```python
from build123d import *

# Parameters (mm, degrees)
SKETCH1_W           = 25.4
SKETCH1_H           = 25.4
SKETCH1_W_2         = 22.225
SKETCH1_H_2         = 22.225
BOSS_EXTRUDE1_DEPTH = 234.95
FILLET1_R           = 2.54
SKETCH2_R           = 3.175
CUT_EXTRUDE1_DEPTH  = 238.560919126
SKETCH3_R           = 1.7
CUT_EXTRUDE2_DEPTH  = 2.54


with BuildPart() as part:
    # Sketch1 → Boss-Extrude1 (new body)
    with BuildSketch(Plane.XY):
        with Locations((-11.559591837, -1.275183673)):
            Rectangle(SKETCH1_W, SKETCH1_H)
        with Locations((-11.559591837, -1.275183673)):
            Rectangle(SKETCH1_W_2, SKETCH1_H_2, mode=Mode.SUBTRACT)
    extrude(amount=BOSS_EXTRUDE1_DEPTH)

    # Fillet1
    fillet1_edges = [part.edges().sort_by_distance(p)[0] for p in [
        (-24.259591837, 11.424816327, 117.475),
        (1.140408163, 11.424816327, 117.475),
        (1.140408163, -13.975183673, 117.475),
        (-24.259591837, -13.975183673, 117.475),
    ]]
    fillet(fillet1_edges, radius=FILLET1_R)

    # Sketch2 → Cut-Extrude1 (cut, through all)
    with BuildSketch(Plane(origin=(0, 11.424816327, 0), x_dir=(1, 0, 0), z_dir=(0, 1, 0))):
        with Locations(Location((-11.559591837, -12.7, 0), (0, 0, 270))):
            Circle(SKETCH2_R)
        with Locations(Location((-11.559591837, -38.1, 0), (0, 0, 270))):
            Circle(SKETCH2_R)
    extrude(amount=-CUT_EXTRUDE1_DEPTH, mode=Mode.SUBTRACT)

    # Sketch3 → Cut-Extrude2 (cut)
    with BuildSketch(Plane(origin=(0, 11.424816327, 0), x_dir=(1, 0, 0), z_dir=(0, 1, 0))):
        with Locations(Location((-6.745071652, -209.51091592, 0), (0, 0, 270))):
            Circle(SKETCH3_R)
        with Locations(Location((-4.172146269, -206.096528614, 0), (0, 0, 270))):
            Circle(SKETCH3_R)
        with Locations(Location((-3.921994623, -221.549522883, 0), (0, 0, 270))):
            Circle(SKETCH3_R)
        with BuildLine():
            Line((-15.016431655, -223.31216962), (-17.859841481, -227.085501905))
            ThreePointArc((-17.859841481, -227.085501905), (-20.240607387, -227.420096733), (-20.575202215, -225.039330826))
            Line((-20.575202215, -225.039330826), (-17.731792389, -221.265998541))
            ThreePointArc((-17.731792389, -221.265998541), (-15.351026483, -220.931403713), (-15.016431655, -223.31216962))
        make_face()
        with BuildLine():
            Line((-18.594632259, -208.581648392), (-17.777811336, -209.185849998))
            ThreePointArc((-17.777811336, -209.185849998), (-17.422050667, -211.563545173), (-19.799745842, -211.919305842))
            Line((-19.799745842, -211.919305842), (-20.616566765, -211.315104237))
            ThreePointArc((-20.616566765, -211.315104237), (-20.972327435, -208.937409062), (-18.594632259, -208.581648392))
        make_face()
    extrude(amount=-CUT_EXTRUDE2_DEPTH, mode=Mode.SUBTRACT)


solid = part.part
```
The listing builds one solid part. Answer for the finished solid, in the listing's coordinates (mm). A direction names the side the tool comes from. Give positions to 0.01 mm unless a question says otherwise; leave off trailing zeros. Order: outer loops, then holes, each group sorted by start corner. A loop starts at its lowest first (then second) coordinate and runs counter-clockwise, first axis right, second up.
Item 1: The part is cut by section C-C, the plane z = 109. Give the vertices of the cut face in (x, y), and give its area (3 significant figures).
From the geometry:
outline: (-24.26, -11.44) arc R2.54 ccw to (-21.72, -13.98) - (-1.4, -13.98) arc R2.54 ccw to (1.14, -11.44) - (1.14, 8.88) arc R2.54 ccw to (-1.4, 11.42) - (-21.72, 11.42) arc R2.54 ccw to (-24.26, 8.88) - close; hole (-22.67, -12.39) - (-0.45, -12.39) - (-0.45, 9.84) - (-22.67, 9.84) - close
area: 146 mm2
Item 2: The part is cut by section B-B, the plane y = -6.25. Give the vertices of the cut face in (x, z), and give its area (3 significant figures).
From the geometry:
outline: (-24.26, 0) - (-22.67, 0) - (-22.67, 234.95) - (-24.26, 234.95) - close; (-0.45, 0) - (1.14, 0) - (1.14, 234.95) - (-0.45, 234.95) - close
area: 746 mm2
Item 3: Given pin 1 Ø5.5 at (x, z) = (-11.56, 12.7) entering from +Y, flat-ended and moving along its own axis, determine where the tip first touches the part or whether it passes through.
From the geometry:
pin 1: passes through
Item 4: The part is cut by section A-A, the plane z = 38.1. Give the vertices of the cut face in (x, y).
From the geometry:
outline: (-24.26, -11.44) arc R2.54 ccw to (-21.72, -13.98) - (-14.73, -13.98) - (-14.73, -12.39) - (-22.67, -12.39) - (-22.67, 9.84) - (-14.73, 9.84) - (-14.73, 11.42) - (-21.72, 11.42) arc R2.54 ccw to (-24.26, 8.88) - close; (-8.38, -13.98) - (-1.4, -13.98) arc R2.54 ccw to (1.14, -11.44) - (1.14, 8.88) arc R2.54 ccw to (-1.4, 11.42) - (-8.38, 11.42) - (-8.38, 9.84) - (-0.45, 9.84) - (-0.45, -12.39) - (-8.38, -12.39) - close
Item 5: Which of the six approach directions +Z, -Z, +X, -X, +Y, -Y give full straight-line access (tool end or side, diameter ignored) to faces 5 (the face through (-12, -12.388, 116)), 6 (the face through (-13.49, -13.17, 35.58))?
From the geometry:
face 5: +Z, -Z
face 6: +Y, -Y
Item 6: Find the intervals of material crossed by probe 1 along X at (y, z) = (6, 100.5); probe 2 along Y at (x, z) = (-19.75, 168.5); probe 3 along X at (y, z) = (10.65, 12.7), in increasing order.
From the geometry:
probe 1: x = -24.26 to -22.67, -0.45 to 1.14
probe 2: y = -13.98 to -12.39, 9.84 to 11.42
probe 3: x = -23.55 to -14.73, -8.38 to 0.43
Item 7: For a pull along X with two mould halves and no side action, classify faces 1 (the face through (-12, 11.425, 116)), 2 (the face through (-13.49, 10.64, 35.58)), 3 (the face through (-13.49, -13.17, 10.18)), 4 (the face through (-24.26, -1, 116)) as pulls with the +X half, pulls with the -X half, needs draft (parallel to the pull), parting line crosses it, or undercut.
From the geometry:
face 1: needs draft
face 2: undercut
face 3: undercut
face 4: pulls with the -X half
